Can you work these out from the model? Positions are in its coordinate system, mm. Face numbers are marked on the shaded views. A direction names the side the tool comes from. Give positions to 0.01 mm unless a question says otherwise; leave off trailing zeros. Write each loop counter-clockwise with the first axis right and the second up, starting at its lowest first coordinate (ties: lowest second). Pieces come first, ordered by that corner, then holes.
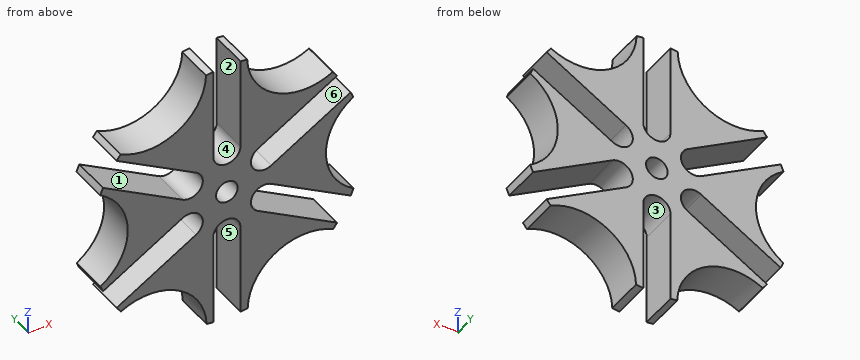
from build123d import *

# Parameters (mm, degrees)
F0_R            = 25
F1_DEPTH        = 7
F3_DEPTH        = 13.3
F3_COPIES_COUNT = 6
F4_R            = 2
F5_DEPTH        = 25


# Not quite as in the source:
# - a pattern or mirror of a feature is missing from the dataset's text; its kind, count and spacing are read off the source's solid


with BuildPart() as f1:
    # F0 (on Front) → F1 (new body)
    with BuildSketch(Plane.XZ):
        Circle(F0_R)
    extrude(amount=F1_DEPTH)

    # F2 (on face) → F3 (cut)
    with BuildSketch(Plane.XZ.offset(7)):
        with BuildLine():
            ThreePointArc((-19.5394295308, 15.5952138046), (-12.5429522443, 21.6257797315), (-3.8342431732, 24.704221892))
            ThreePointArc((-3.8342431732, 24.704221892), (-3.8311679177, 24.8520967356), (-3.8301427668, 25))
            ThreePointArc((-3.8301427668, 25), (-19.9806869892, 34.1546667609), (-19.5394295308, 15.5952138046))
        make_face()
        with BuildLine():
            ThreePointArc((-19.5394295308, 15.5952138046), (-9.1467396108, 15.7702407083), (-3.8342431732, 24.704221892))
            ThreePointArc((-3.8342431732, 24.704221892), (-12.5429522443, 21.6257797315), (-19.5394295308, 15.5952138046))
        make_face()
        with BuildLine():
            ThreePointArc((2.4968730444, 24.875), (2.4992181388, 24.9374804474), (2.5, 25))
            ThreePointArc((2.5, 25), (0, 27.5), (-2.5, 25))
            ThreePointArc((-2.5, 25), (-2.4992181388, 24.9374804474), (-2.4968730444, 24.875))
            ThreePointArc((-2.4968730444, 24.875), (0, 25), (2.4968730444, 24.875))
        make_face()
        with BuildLine():
            ThreePointArc((-2.4968730444, 24.875), (0, 22.5), (2.4968730444, 24.875))
            ThreePointArc((2.4968730444, 24.875), (0, 25), (-2.4968730444, 24.875))
        make_face()
        with BuildLine():
            ThreePointArc((2.5, 24.8746859277), (2.4984365271, 24.874843013), (2.4968730444, 24.875))
            ThreePointArc((2.4968730444, 24.875), (0, 22.5), (-2.4968730444, 24.875))
            ThreePointArc((-2.4968730444, 24.875), (-2.4984365271, 24.874843013), (-2.5, 24.8746859277))
            Line((-2.5, 24.8746859277), (-2.5, 8))
            ThreePointArc((-2.5, 8), (0, 10.5), (2.5, 8))
            Line((2.5, 8), (2.5, 24.8746859277))
        make_face()
        with BuildLine():
            ThreePointArc((-2.5, 8), (0, 5.5), (2.5, 8))
            ThreePointArc((2.5, 8), (0, 10.5), (-2.5, 8))
        make_face()
    f3 = extrude(amount=-F3_DEPTH, mode=Mode.SUBTRACT)

    # F3_copies: F3 ×6 about axis
    f3_copies_axis = Axis((0, 0, 0), (0, 1, 0))
    for i in range(1, F3_COPIES_COUNT):
        add(f3.rotate(f3_copies_axis, i * 360 / F3_COPIES_COUNT), mode=Mode.SUBTRACT)

    # F4 (on face) → F5 (cut)
    with BuildSketch(Plane.XZ.offset(7)):
        Circle(F4_R)
    extrude(amount=-F5_DEPTH, mode=Mode.SUBTRACT)


solid = f1.part
(1) If I drill on L1, parallel to Z at x = 0, y = -3; L2, parallel to Z at x = -12, y = -0.5; L3, parallel to Z at x = -9, y = -1.5, over which ranges is the centre line in solid material (lowest first)?
Returned:
L1: z = -5.5 to -2, 2 to 5.5
L2: z = -14.66 to -9.81, -4.04 to 4.04, 9.81 to 14.63
L3: z = -15.86 to -8.08, -2.31 to 2.31, 8.08 to 15.86
(2) Imagine slicing it at D-D, the plane x = 7. Write out the boundary of the cut face in (y, z), plus the area to 3 significant figures.
Returned:
outline: (-7, -17.41) - (0, -17.41) - (0, -6.93) - (-7, -6.93) - close; (-7, -1.5) - (0, -1.5) - (0, 1.5) - (-7, 1.5) - close; (-7, 6.93) - (0, 6.93) - (0, 17.37) - (-7, 17.37) - close
area: 167 mm2
(3) If we mould it in two halves opening along Z, with no side actions, what happens to the marked faces 1, 2 and 3? For each: +Z half, -Z half, draft (parallel to the pull), parting line (faces both ways), or undercut.
Returned:
face 1: undercut
face 2: draft
face 3: -Z half
(4) Imagine slicing it at B-B, the plane z = 0. Write out the boundary of the cut face in (x, y).
Returned:
outline: (-18.23, -7) - (-2, -7) - (-2, 0) - (-18.23, 0) - close; (2, -7) - (18.23, -7) - (18.23, 0) - (2, 0) - close
(5) Imagine slicing it at C-C, the plane x = 0. Write out the boundary of the cut face in (y, z), plus the area to 3 significant figures.
Returned:
outline: (-7, -5.5) - (0, -5.5) - (0, -2) - (-7, -2) - close; (-7, 2) - (0, 2) - (0, 5.5) - (-7, 5.5) - close
area: 49.0 mm2
(6) Will these pins go through, and if not, where does the flat tip stop? P1, Ø1, axis at x = -11, y = -6, coming from the +Z side; P2, Ø4, axis at y = -1, z = 4, coming from the +X side; P3, Ø3.5, axis at y = -5, z = -15.5, coming from the -X side; P4, Ø3.5, axis at x = 0, z = 0, coming from the -Y side.
Returned:
P1: stops at z = 15.11
P2: stops at x = 20.04
P3: stops at x = -20.29
P4: passes through
(7) Imagine slicing it at A-A, the plane x = 17.5. Write out the boundary of the cut face in (y, z), plus the area to 3 significant figures.
Returned:
outline: (-7, -14.76) - (0, -14.76) - (0, -12.99) - (-7, -12.99) - close; (-7, -7.22) - (0, -7.22) - (0, 7.22) - (-7, 7.22) - close; (-7, 12.99) - (0, 12.99) - (0, 14.85) - (-7, 14.85) - close
area: 126 mm2
(8) For the marked faces 4, 5 and 6, which set-ups out of +Z, -Z, +X, -X, +Y, -Y let a thin tool reach every point of the face, with its end or its side?
Returned:
face 4: +Z, +Y, -Y
face 5: -Z, +Y, -Y
face 6: +Y, -Y
